```python
from build123d import *

# Parameters (mm, degrees)
SKETCH_1_W          = 17
SKETCH_1_H          = 20
EXTRUDE_1_DEPTH     = 3
SKETCH_2_W          = 17
SKETCH_2_H          = 3
EXTRUDE_2_DEPTH     = 17
CUT_EXTRUDE_1_DEPTH = 17
EXTRUDE_3_DEPTH     = 2.25
EXTRUDE_4_DEPTH     = 2.25


with BuildPart() as part:
    # Эскиз1 → Бобышка-Вытянуть1 (new body)
    with BuildSketch(Plane.XY):
        with Locations((-20.775029161, -4.314630229)):
            Rectangle(SKETCH_1_W, SKETCH_1_H)
        with BuildLine():
            Line((-17.775029161, -3.314630229), (-17.775029161, -6.314630229))
            ThreePointArc((-17.775029161, -6.314630229), (-20.775029161, -9.314630229), (-23.775029161, -6.314630229))
            Line((-23.775029161, -6.314630229), (-23.775029161, -3.314630229))
            ThreePointArc((-23.775029161, -3.314630229), (-20.775029161, -0.314630229), (-17.775029161, -3.314630229))
        make_face(mode=Mode.SUBTRACT)
    extrude(amount=EXTRUDE_1_DEPTH)

    # Эскиз2 → Бобышка-Вытянуть2 (add)
    with BuildSketch(Plane.XY.offset(3)):
        with Locations((-20.775029161, 4.185369771)):
            Rectangle(SKETCH_2_W, SKETCH_2_H)
    extrude(amount=EXTRUDE_2_DEPTH)

    # Эскиз3 → Вырез-Вытянуть1 (cut)
    with BuildSketch(Plane.XZ.offset(-2.685369771)):
        with BuildLine():
            Line((-17.775029161, 12), (-17.775029161, 9))
            ThreePointArc((-17.775029161, 9), (-20.775029161, 6), (-23.775029161, 9))
            Line((-23.775029161, 9), (-23.775029161, 12))
            ThreePointArc((-23.775029161, 12), (-20.775029161, 15), (-17.775029161, 12))
        make_face()
    extrude(amount=-CUT_EXTRUDE_1_DEPTH, mode=Mode.SUBTRACT)

    # Эскиз4 → Бобышка-Вытянуть3 (add)
    with BuildSketch(Plane.ZY.offset(29.275029161)):
        Polygon((20, 2.685369771), (3, 2.685369771), (3, -14.314630229), align=None)
    extrude(amount=-EXTRUDE_3_DEPTH)

    # Эскиз5 → Бобышка-Вытянуть4 (add)
    with BuildSketch(Plane(origin=(-12.275029161, 0, 0), x_dir=(0, 0, -1), z_dir=(1, 0, 0))):
        Polygon((-3, -14.314630229), (-3, 2.685369771), (-20, 2.685369771), align=None)
    extrude(amount=-EXTRUDE_4_DEPTH)


solid = part.part
```
Geometry check sheet. Reference: the model listing, model coordinates, mm. A direction names the side the tool comes from. Round coordinates to 2 decimals unless told otherwise and drop trailing zeros. Order: outer loops, then holes, each group sorted by start corner. A loop starts at its lowest first (then second) coordinate and runs counter-clockwise, first axis right, second up. Notation, with made-up numbers: (79, 87.25) -> (102, 87.25) arc R36 ccw to (102, 126.25) -> close; hole circle Ø6 at (13.25, 82.25). An arc over 180 degrees is marked (long way). Return JSON: item names as keys, results as strings. Group by question number.
Q1. Material ranges on probe 1 along X at (y, z) = (-3.75, 13.5); probe 2 along Z at (x, y) = (-24.5, -9); probe 3 along Y at (x, z) = (-17.25, 14.5), recorded low to high. Write a range as from..to.
Q2. Tool access check on faces 4 (the cylindrical face through (-20.709, -9.314, 1.479)), 5 (the flat face through (-24, -8, 3)), 6 (the flat face through (-17.775, 4, 11)). Record the directions out of +Z, -Z, +X, -X, +Y, -Y that give a thin tool (end or side, any length) a straight path to the whole face; none if there is none.
Q3. Section check D-D, the plane y = -10. Record the boundary of the cut face in (x, z).
Q4. Release check for a two-part mould opening along Y. For faces 1 (the flat face through (-14.525, -2, 8)), 2 (the flat face through (-23.775, -5, 1)), 3 (the flat face through (-21, -14.315, 1)) record: released by +Y, released by -Y, zero draft, split by the parting line, or undercut.
Q5. Section check B-B, the plane x = -20.75. Record the boundary of the cut face in (y, z), plus the area to 3 significant figures.
Q6. Section check C-C, the plane y = -4. Record the boundary of the cut face in (x, z), plus the area to 3 significant figures.
Q7. Section check A-A, the plane z = 10.25. Record the boundary of the cut face in (x, y).
Q8. Gauge pin test, flat end, axial feed: pin 1 (10 mm diameter, centred on x = -17.5, z = 6, fed in from -Y). Record the tip position at first contact, or that the pin passes through.
Numbers:
{
 "1": {"probe 1": "-29.28..-27.03, -14.53..-12.28", "probe 2": "0..3", "probe 3": "2.69..5.69"},
 "2": {"face 4": "+Z, -Z", "face 5": "+Z, -Y", "face 6": "+Y, -Y"},
 "3": {"outline": "(-29.28, 0) -> (-12.28, 0) -> (-12.28, 7.31) -> (-14.53, 7.31) -> (-14.53, 3) -> (-27.03, 3) -> (-27.03, 7.31) -> (-29.28, 7.31) -> close"},
 "4": {"face 1": "zero draft", "face 2": "undercut", "face 3": "released by -Y"},
 "5": {"outline": "(-14.31, 0) -> (-9.31, 0) -> (-9.31, 3) -> (-14.31, 3) -> close; (-0.31, 0) -> (5.69, 0) -> (5.69, 6) -> (2.69, 6) -> (2.69, 3) -> (-0.31, 3) -> close; (2.69, 15) -> (5.69, 15) -> (5.69, 20) -> (2.69, 20) -> close", "area": "57.0 mm^2"},
 "6": {"outline": "(-29.28, 0) -> (-23.78, 0) -> (-23.78, 3) -> (-27.03, 3) -> (-27.03, 13.31) -> (-29.28, 13.31) -> close; (-17.78, 0) -> (-12.28, 0) -> (-12.28, 13.31) -> (-14.53, 13.31) -> (-14.53, 3) -> (-17.78, 3) -> close", "area": "79.4 mm^2"},
 "7": {"outline": "(-29.28, -7.06) -> (-27.03, -7.06) -> (-27.03, 2.69) -> (-23.78, 2.69) -> (-23.78, 5.69) -> (-29.28, 5.69) -> close; (-17.78, 2.69) -> (-14.53, 2.69) -> (-14.53, -7.06) -> (-12.28, -7.06) -> (-12.28, 5.69) -> (-17.78, 5.69) -> close"},
 "8": {"pin 1": "y = -14.31"}
}
